Could you check a few things on this model? Use its own coordinates, in mm. A direction names the side the tool comes from. Coordinates: 2 decimals unless noted, no trailing zeros. Loops run counter-clockwise (first coordinate to the right, second up) from the corner with the lowest first, then second, coordinate; pieces in that order, holes last. Notation, with made-up numbers: (-39, 2) - (-25, 2) arc R7 cw to (-25, 9) - close; hole circle Ø9 at (11, 53.5). An arc over 180 degrees is marked (long way). One line per item, written item: value. Start each with the question number.
(1) I'm going to push flat-ended pins straight in: P1, Ø8, axis at x = -13.5, z = -11.5, coming from the +Y side; P2, Ø4, axis at y = 13.5, z = -13, coming from the +X side; P3, Ø12, axis at x = 25.5, z = -1.5, coming from the -Y side; P4, Ø16, axis at y = 36.8, z = 0, coming from the -X side. Where does each tip first touch, or does it pass through?
(2) If we section it at D-D on x = 25.5: Write out the boundary of the cut face in (y, z) (3 decimals), then the cut area to 3 significant figures.
(3) If I drill on line 1 along Z through (x, y) = (0, 9) (3 decimals); line 2 along X through (y, z) = (22, 0) (3 decimals), over which ranges is the centre line in solid material (lowest first)? Write a range as from..to.
(4) On a 3-axis mill with a long thin cutter (end or side, diameter ignored), from which of +Z, -Z, +X, -X, +Y, -Y can I reach the whole of each face in a straight line? I mean faces 5 (the face through (-1, 0, 14)), 6 (the face through (12.16, 14.05, -11.15)). Say none if no direction works.
(5) If we mould it in two halves opening along Z, with no side actions, what happens to faces 1 (the face through (0.512, 50.012, 1.735)), 2 (the face through (-36.57, 38, 14)), 3 (the face through (0.512, 52.538, 4.956)), 4 (the face through (-1.735, 14.054, 13.212))? For each: pulls with the +Z half, pulls with the -Z half, needs draft (parallel to the pull), parting line crosses it, or undercut.
(6) If we section it at B-B on y = 36: Write out the boundary of the cut face in (x, z) (3 decimals), then the cut area to 3 significant figures.
(7) If we section it at A-A on z = 0: Write out the boundary of the cut face in (x, y) (3 decimals), then the cut area to 3 significant figures.
(8) If we section it at C-C on x = 0: Write out the boundary of the cut face in (y, z) (3 decimals), then the cut area to 3 significant figures.
Autodesk Inventor part; units mm, degrees
ref_plane "YZ Plane" through (0, 0, 0) normal (1, 0, 0) x (0, 1, 0)
ref_plane "XZ Plane" through (0, 0, 0) normal (0, 1, 0) x (-1, 0, 0)
ref_plane "XY Plane" through (0, 0, 0) normal (0, 0, 1) x (1, 0, 0)
sketch "Boceto2" plane through (0, 0, 0) normal (0, 1, 0) x (-1, 0, 0)
  circle A0 centre (0, 0) radius 16.5
  dimension "d0" = 33
extrude "Extrusión1" add sketch "Boceto2" along normal blind 36.8
sketch "Boceto3" plane through (0, 0, 0) normal (1, 0, 0) x (0, 1, 0)
  line L0 (0, 0) -> (36.8, 0)
  line L1 (36.8, -16.5) -> (36.8, 16.5)
  circle A0 centre (36.8, 0) radius 16.5
extrude "Extrusión2" add sketch "Boceto3" along normal mid plane 73.14
sketch "Boceto4" plane through (36.57, 36.8, 0) normal (1, 0, 0) x (0, 0, -1)
  circle A0 centre (0, 0) radius 13.325
  point P0 (0, -36.8)
  dimension "d5" = 26.65
extrude "Extrusión3" cut sketch "Boceto4" against normal blind 73.14
sketch "Boceto5" plane through (0, 0, 0) normal (0, -1, 0) x (1, 0, 0)
  circle A0 centre (0, 0) radius 13.325
  dimension "d8" = 26.65
extrude "Extrusión4" cut sketch "Boceto5" against normal up to surface
properties part number "T" material "PVC, no plastificado"
Values:
1. P1: stops at y = 51.5
1. P2: stops at x = 12.3
1. P3: stops at y = 20.3
1. P4: passes through
2. outline: circle Ø33 at (36.8, 0); hole circle Ø26.65 at (36.8, 0)
2. area: 297 mm2
3. line 1: z = -16.5..-13.325, 13.325..16.5
3. line 2: x = -36.57..-13.325, 13.325..36.57
4. face 5: +Z, -Z, +X, -X, -Y
4. face 6: -Y
5. face 1: undercut
5. face 2: needs draft
5. face 3: parting line crosses it
5. face 4: undercut
6. outline: (-36.57, -16.481) - (-0.8, -16.481) arc R16.5 ccw to (0.8, -16.481) - (36.57, -16.481) - (36.57, -13.301) - (0.8, -13.301) arc R13.325 cw to (-0.8, -13.301) - (-36.57, -13.301) - close; (-36.57, 13.301) - (-0.8, 13.301) arc R13.325 cw to (0.8, 13.301) - (36.57, 13.301) - (36.57, 16.481) - (0.8, 16.481) arc R16.5 ccw to (-0.8, 16.481) - (-36.57, 16.481) - close
6. area: 465 mm2
7. outline: (-36.57, 20.3) - (-16.5, 20.3) - (-16.5, 0) - (-13.325, 0) - (-13.325, 23.475) - (-36.57, 23.475) - close; (-36.57, 50.125) - (36.57, 50.125) - (36.57, 53.3) - (-36.57, 53.3) - close; (13.325, 0) - (16.5, 0) - (16.5, 20.3) - (36.57, 20.3) - (36.57, 23.475) - (13.325, 23.475) - close
7. area: 509 mm2
8. outline: (0, -16.5) - (36.8, -16.5) arc R16.5 ccw to (36.8, 16.5) - (0, 16.5) - (0, 13.325) - (36.8, 13.325) arc R13.325 cw to (36.8, -13.325) - (0, -13.325) - close
8. area: 382 mm2
